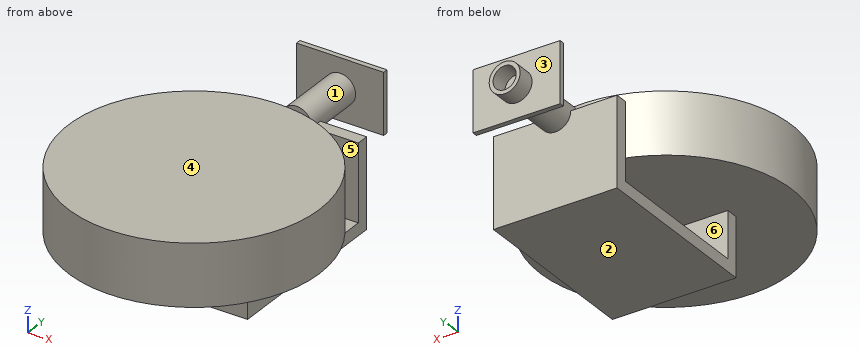
from build123d import *

# Parameters (mm, degrees)
SKETCH1_R                = 101.6
BOSS_EXTRUDE1_DEPTH      = 50
SKETCH4_W                = 12.5
SKETCH4_H                = 71.371504998
EXTRUDE_THIN1_DEPTH      = 50
EXTRUDE_THIN1_DEPTH_BACK = 50
SKETCH5_R                = 9.366113587
CUT_EXTRUDE1_DEPTH       = 50
SKETCH6_W                = 70.465682624
SKETCH6_H                = 49.159233517
BOSS_EXTRUDE2_DEPTH      = 4


with BuildPart() as part:
    # Sketch1 → Boss-Extrude1 (new body)
    with BuildSketch(Plane.XY):
        Circle(SKETCH1_R)
    extrude(amount=BOSS_EXTRUDE1_DEPTH)



with BuildPart() as body_2:
    # Sketch4 → Revolve-Thin1 (revolve)
    with BuildSketch(Plane(origin=(0, 0, 0), x_dir=(0, 0, -1), z_dir=(1, 0, 0)), mode=Mode.PRIVATE) as revolve_thin1_sk:
        with Locations((-30.829616759, 159.903955702)):
            Rectangle(SKETCH4_W, SKETCH4_H)
    revolve(revolve_thin1_sk.sketch.rotate(Axis((0, 124.218203203, 24.579616759), (0, 1, 0)), 180), axis=Axis((0, 124.218203203, 24.579616759), (0, 1, 0)))


with BuildPart() as part_1:
    add(part.part)

    add(body_2.part)  # Extrude-Thin1 merges body 2
    # Sketch3 → Extrude-Thin1 (add, two sides: drawn at the far end of the back side and taken through both)
    with BuildSketch(Plane(origin=(0, 0, 0), x_dir=(0, 0, -1), z_dir=(1, 0, 0)).offset(-EXTRUDE_THIN1_DEPTH_BACK)):
        Polygon((-24.579616759, 0), (37.637102953, 0), (37.637102953, 124.218203203), (-24.579616759, 124.218203203), (-24.579616759, 134.218203203), (47.637102953, 134.218203203), (47.637102953, -10), (-24.579616759, -10), align=None)
    extrude(amount=EXTRUDE_THIN1_DEPTH + EXTRUDE_THIN1_DEPTH_BACK)

    # Sketch5 → Cut-Extrude1 (cut)
    with BuildSketch(Plane(origin=(0, 195.589708201, 0), x_dir=(1, 0, 0), z_dir=(0, 1, 0))):
        with Locations(Location((0, -24.579616759, 0), (0, 0, 270))):
            Circle(SKETCH5_R)
    extrude(amount=-CUT_EXTRUDE1_DEPTH, mode=Mode.SUBTRACT)

    # Sketch6 → Boss-Extrude2 (add)
    with BuildSketch(Plane(origin=(0, 177.126182074, 0), x_dir=(1, 0, 0), z_dir=(0, 1, 0))):
        with Locations((0, -24.579616759)):
            Rectangle(SKETCH6_W, SKETCH6_H)
    extrude(amount=BOSS_EXTRUDE2_DEPTH)


solid = part_1.part
Work out the finished part from the listing and answer in its coordinate system (mm). Face numbers are marked on the shaded views. A direction names the side the tool comes from. Coordinates: 2 decimals unless noted, no trailing zeros. Write each loop counter-clockwise with the first axis right and the second up, starting at its lowest first coordinate (ties: lowest second). Pieces come first, ordered by that corner, then holes. Notation, with made-up numbers: M -24.5,24 L 33.5,24 A12 ccw 33.5,30 Z; hole C 84.5,-19.75 d8. An arc over 180 degrees is marked long. Answer as CSV lines item,"result". Start each with the question number.
Item 1: Section D-D on y = -46 is taken. Write down the section's boundary in (x, z), and give its area (3 significant figures).
Item 2: Consider L1, parallel to Y at x = 15.5, z = -36; L2, parallel to Z at x = -21.5, y = 47.5; L3, parallel to Z at x = 76, y = -5.5. Determine where each line is inside the solid, lowest interval first.
Item 3: Section A-A on z = -8.5 is taken. Write down the section's boundary in (x, y).
Item 4: Determine the mould class of the marked faces 3, 4, 5 and 6 for opening direction Y: released by +Y, released by -Y, zero draft, split by the parting line, or undercut.
Item 5: Flat-ended cylindrical pins translate along their axes: P1, Ø8, axis at y = 22.5, z = 5, coming from the -X side; P2, Ø9.5, axis at x = 2.5, z = 26, coming from the +Y side; P3, Ø10, axis at y = -49, z = 34.5, coming from the +X side; P4, Ø4, axis at x = -53, z = -21, coming from the +Y side. Find the tip coordinate at first contact, or state that the pin passes through.
Item 6: Section C-C on z = 21 is taken. Write down the section's boundary in (x, y), and give its area (3 significant figures).
Item 7: A tool of negligible diameter and unlimited length cuts with its end or side. For the marked faces 1 and 2, from which of +Z, -Z, +X, -X, +Y, -Y can it reach the whole face along a straight path? Write none if from no direction.
Checks:
1,outline,"M -90.59,0 L 90.59,0 L 90.59,50 L -90.59,50 Z"
1,area,"9,060 mm²"
2,L1,"y = -10 to 0, 124.22 to 134.22"
2,L2,"z = -47.64 to -37.64, 0 to 50"
2,L3,"z = 0 to 50"
3,outline,"M -50,-10 L 50,-10 L 50,0 L -50,0 Z; M -50,124.22 L 50,124.22 L 50,134.22 L -50,134.22 Z"
4,face 3,"released by +Y"
4,face 4,"zero draft"
4,face 5,"undercut"
4,face 6,"undercut"
5,P1,"stops at x = -99.9"
5,P2,"stops at y = 181.13"
5,P3,"stops at x = 91.58"
5,P4,"passes through"
6,outline,"C 0,0 d203.2; M -50,124.22 L 50,124.22 L 50,134.22 L 11.98,134.22 L 11.98,177.13 L 35.23,177.13 L 35.23,181.13 L 11.98,181.13 L 11.98,195.59 L 8.66,195.59 L 8.66,181.13 L -8.66,181.13 L -8.66,195.59 L -11.98,195.59 L -11.98,181.13 L -35.23,181.13 L -35.23,177.13 L -11.98,177.13 L -11.98,134.22 L -50,134.22 Z; hole M -8.66,145.59 L 8.66,145.59 L 8.66,177.13 L -8.66,177.13 Z"
6,area,"34,300 mm²"
7,face 1,"none"
7,face 2,"-Z, +X, -X, +Y, -Y"
